Autodesk Fusion 360 part; units mm, degrees
sketch "Sketch1" plane through (0, 0, 0) normal (0, 0, 1) x (1, 0, 0)
  line L0 (0, 0) -> (40, 0)
  line L1 (40, 0) -> (40, 30)
  line L2 (40, 30) -> (0, 30)
  line L3 (0, 30) -> (0, 0)
  dimension "d1" = 40
  dimension "d2" = 30
extrude "Extrude1" add sketch "Sketch1" along normal blind 1.2
sketch "Sketch2" plane through (0, 0, 1.2) normal (0, 0, 1) x (-1, 0, 0)
  line L0 (0, -30) -> (0, 0)
  line L1 (0, 0) -> (-40, 0)
  line L2 (-40, 0) -> (-40, -30)
  line L3 (-40, -30) -> (0, -30)
sketch "Sketch3" plane through (0, 0, 1.2) normal (0, 0, 1) x (-1, 0, 0)
sketch "Sketch4" plane through (0, 0, 1.2) normal (0, 0, 1) x (-1, 0, 0)
  line L0 (-40, 0) -> (-40, -30)
  line L1 (-40, -30) -> (0, -30)
  circle A0 centre (-2.75, -26.5) radius 1
  circle A1 centre (-2.75, -3.5) radius 1
  circle A2 centre (-37.25, -26.5) radius 1
  circle A3 centre (-37.0314, -3.5) radius 1
  point P0 (-20, -30)
  point P1 (-40, -15)
  point P2 (-37.25, -26.5)
  point P3 (-37.0314, -3.5)
  point P4 (-2.75, -26.5)
  point P5 (-2.75, -3.5)
  dimension "d8" = 11.5
  dimension "d9" = 17.25
  dimension "d10" = 23
  dimension "d11" = 34.5
  dimension "d12" = 2
  dimension "d13" = 2
  dimension "d14" = 2
  dimension "d15" = 2
hole "Hole1" at (2.75, 3.5, 1.2) at (37.0314, 3.5, 1.2) at (37.25, 26.5, 1.2) at (2.75, 26.5, 1.2) direction (0, 0, -1) diameter 2 depth 1.5 tip angle 180
The listing builds one solid part. Answer for the finished solid, in the listing's coordinates (mm). Coordinates: 2 decimals unless noted, no trailing zeros. Write each loop counter-clockwise with the first axis right and the second up, starting at its lowest first coordinate (ties: lowest second). Pieces come first, ordered by that corner, then holes. Notation, with made-up numbers: M 0,89 L 27,89 A17 ccw 27,108 Z; hole C 48,69.5 d2. An arc over 180 degrees is marked long. Use one line per item in the form item = value.
Item 1: The mould has two halves that part along X. Classify faces 1 (the face through (0, 15, 1)), 2 (the face through (2.7, 27.5, 0.6)), 3 (the face through (20, 30, 1)): released by +X, released by -X, zero draft, split by the parting line, or undercut.
Model answer:
face_1 = released by -X
face_2 = undercut
face_3 = zero draft
Item 2: Find section A-A, the plane y = 26.5. Give the vertices of the cut face in (x, z), plus the area to 3 significant figures.
Model answer:
outline = M 0,0 L 1.75,0 L 1.75,1.2 L 0,1.2 Z; M 3.75,0 L 36.25,0 L 36.25,1.2 L 3.75,1.2 Z; M 38.25,0 L 40,0 L 40,1.2 L 38.25,1.2 Z
area = 43.2 mm2
Item 3: Find the intervals of material crossed by probe 1 along X at (y, z) = (3.5, 0.4); probe 2 along X at (y, z) = (26.5, 0.65), in increasing order.
Model answer:
probe_1 = 0 to 1.75, 3.75 to 36.03, 38.03 to 40
probe_2 = 0 to 1.75, 3.75 to 36.25, 38.25 to 40
Item 4: Find section B-B, the plane x = 2.75. Give the vertices of the cut face in (y, z), plus the area to 3 significant figures.
Model answer:
outline = M 0,0 L 2.5,0 L 2.5,1.2 L 0,1.2 Z; M 4.5,0 L 25.5,0 L 25.5,1.2 L 4.5,1.2 Z; M 27.5,0 L 30,0 L 30,1.2 L 27.5,1.2 Z
area = 31.2 mm2
